Autodesk Inventor part; units mm, degrees
ref_plane "YZ Plane" through (0, 0, 0) normal (1, 0, 0) x (0, 1, 0)
ref_plane "XZ Plane" through (0, 0, 0) normal (0, 1, 0) x (-1, 0, 0)
ref_plane "XY Plane" through (0, 0, 0) normal (0, 0, 1) x (1, 0, 0)
sketch "Esboço1" plane through (0, 0, 0) normal (0, 0, 1) x (1, 0, 0)
  circle A0 centre (0, 0) radius 11
  dimension "d0" = 22
extrude "Extrusão1" add sketch "Esboço1" along normal blind 3.5
sketch "Esboço2" plane through (0, 0, 3.5) normal (0, 0, 1) x (1, 0, 0)
  circle A0 centre (0, 0) radius 5
  dimension "d3" = 10
extrude "Extrusão2" add sketch "Esboço2" along normal blind 1.5
sketch "Esboço3" plane through (0, 0, 0) normal (0, 0, -1) x (-1, 0, 0)
  circle A0 centre (0, 0) radius 5
  dimension "d6" = 10
extrude "Extrusão3" add sketch "Esboço3" along normal blind 10
sketch "Esboço4" plane through (0, 0, 3.5) normal (0, 0, 1) x (1, 0, 0)
  circle A0 centre (0, 0) radius 8 construction
  circle A1 centre (-8, 0) radius 1 construction
  circle A2 centre (0, -8) radius 1 construction
  circle A3 centre (0, 0) radius 8 construction
  circle A4 centre (8, 0) radius 1 construction
  circle A5 centre (0, 0) radius 8 construction
  circle A6 centre (0, 8) radius 1 construction
  circle A7 centre (0, 0) radius 8 construction
  dimension "d9" = 16
  dimension "d10" = 2
  dimension "d13" = 360
hole "Furo1" at (-8, 0, 3.5) at (0, -8, 3.5) at (8, 0, 3.5) at (0, 8, 3.5) direction (0, 0, -1) diameter 3.5 end through all
fillet "Arredondamento1" radius 0.3 4 edges at (-11, 0, 3.5) (-11, 0, 0) (5, 0, -10) (-5, 0, 5)
sketch "Esboço5" plane through (0, 0, 5) normal (0, 0, 1) x (1, 0, 0)
  circle A0 centre (0, 0) radius 1.5 construction
  dimension "d23" = 3
hole "Furo2" at (0, 0, 5) direction (0, 0, -1) diameter 6.5 end through all
properties part number "CastanhaTR8"
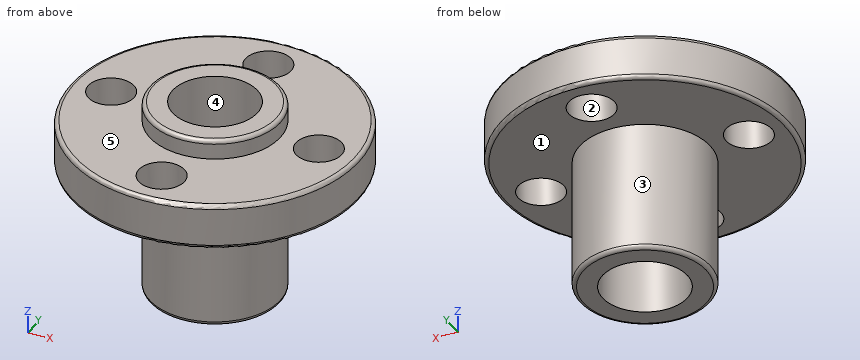
Design review of the part built by this model. Coordinates are the model's own, in mm. Face numbers are marked on the shaded views. A direction names the side the tool comes from. Give positions to 0.01 mm unless a question says otherwise; leave off trailing zeros. Loops run counter-clockwise (first coordinate to the right, second up) from the corner with the lowest first, then second, coordinate; pieces in that order, holes last. Notation, with made-up numbers: (-18, 86.5) - (12, 86.5) arc R36 ccw to (12, 120.5) - close; hole circle Ø6 at (24.25, -40). An arc over 180 degrees is marked (long way). Use CSV: the item, a comma, the result in double quotes. Start each with the question number.
1. Insertion check: P1, Ø8, axis at x = 8.5, y = 7, coming from the +Z side; P2, Ø4.5, axis at x = 0, y = -8, coming from the -Z side; P3, Ø1, axis at y = 4, z = -6, coming from the -X side. Each pin has a flat end and moves straight along its axis. Give the tip position at first contact, or say it passes through.
2. Draft analysis for pull direction X (two halves, no side actions). For the marked faces 1, 2 and 3, state which applies: released by +X, released by -X, zero draft, split by the parting line, or undercut.
3. Add section A-A (x = 0). Count the separate pieces of the cut face and the enclosed holes in it, plus the area to 3 significant figures.
4. Add section C-C (z = -1). State the section outline as (x, y) points, plus the area to 3 significant figures.
5. Machinability: for the marked faces 4 and 5, which of the approach directions +Z, -Z, +X, -X, +Y, -Y give a long, thin tool a straight path to every point of the face, cutting with its end or side? Answer none if there is none.
6. Wall thickness on L1, parallel to Y at x = 0, z = 1.85; L2, parallel to Y at x = 0, z = -4.75; L3, parallel to Z at x = -3.75, y = -9.75: over which ranges is each line inside the solid? List them lowest first.
Results found:
1,P1,"stops at z = 3.5"
1,P2,"stops at z = 0"
1,P3,"stops at x = -3.57"
2,face 1,"zero draft"
2,face 2,"undercut"
2,face 3,"split by the parting line"
3,separate pieces,"4"
3,enclosed holes,"0"
3,area,"69.8 mm²"
4,outline,"circle Ø10 at (0, 0); hole circle Ø6.5 at (0, 0)"
4,area,"45.4 mm²"
5,face 4,"+Z, -Z"
5,face 5,"+Z"
6,L1,"y = -11 to -9.75, -6.25 to -3.25, 3.25 to 6.25, 9.75 to 11"
6,L2,"y = -5 to -3.25, 3.25 to 5"
6,L3,"z = 0 to 3.5"
